```python
from build123d import *

# Parameters (mm, degrees)
F1_DEPTH = 50.8
F3_DEPTH = 45.72
F4_R     = 5.08


with BuildPart() as f1:
    # F0 (on Top) → F1 (new body)
    with BuildSketch(Plane.XY):
        Polygon((23.324189, 60.191778), (-32.517433, 55.764545), (-63.872765, 9.345472), (-47.130602, -44.110932), (5.101866, -64.350904), (53.492524, -36.133333), (61.602221, 19.293375), align=None)
    extrude(amount=F1_DEPTH)

    # F2 (on face) → F3 (cut)
    with BuildSketch(Plane.XY.offset(50.8)):
        Polygon((21.136437, 56.987757), (-31.37647, 52.056417), (-60.262255, 7.925533), (-43.769332, -42.173439), (5.68279, -60.514951), (50.855655, -33.287471), (57.733175, 19.006154), align=None)
    extrude(amount=-F3_DEPTH, mode=Mode.SUBTRACT)

    # F4
    f4_edges = [f1.edges().sort_by_distance(p)[0] for p in [
        (-63.872765, 9.345472, 25.4),
        (-32.517433, 55.764545, 25.4),
        (23.324189, 60.191778, 25.4),
        (61.602221, 19.293375, 25.4),
        (53.492524, -36.133333, 25.4),
        (-47.130602, -44.110932, 25.4),
        (5.101866, -64.350904, 25.4),
    ]]
    fillet(f4_edges, radius=F4_R)


solid = f1.part
```
Design review of the part built by this model. Coordinates are the model's own, in mm. A direction names the side the tool comes from. Give positions to 0.01 mm unless a question says otherwise; leave off trailing zeros. Write each loop counter-clockwise with the first axis right and the second up, starting at its lowest first coordinate (ties: lowest second). Pieces come first, ordered by that corner, then holes. Notation, with made-up numbers: (33, -10) - (53, -10) arc R34 ccw to (53, 27) - close; hole circle Ø4 at (63.5, 89). An arc over 180 degrees is marked (long way). Return JSON: item names as keys, results as strings. Group by question number.
(1) We need section A-A, the plane z = 11. Give the boundary of the cut face in (x, y), then the cut area to 3 significant figures.
(2) We need section B-B, the plane x = -28.5. Give the boundary of the cut face in (y, z), then the cut area to 3 significant figures.
(3) We need section C-C, the plane y = 49. Give the boundary of the cut face in (x, z).
(4) Machinability: for faces 5 (the flat face through (-47.995, 32.852, 25.044)), 6 (the flat face through (-2, -1, 5.08)), which of the approach directions +Z, -Z, +X, -X, +Y, -Y give a long, thin tool a straight path to every point of the face, cutting with its end or side? Answer none if there is none.
(5) To check wall thickness, follow probe 1 along X at (y, z) = (-27.5, 10); probe 2 along Z at (x, y) = (7.5, -21); probe 3 along Y at (x, z) = (41.5, 15.5). State the ranges of each line that lie inside material, in increasing order.
(6) Insertion check: pin 1 (6 mm diameter, centred on y = 8.5, z = 35, fed in from +X); pin 2 (10 mm diameter, centred on y = 10, z = 21.5, fed in from +X); pin 3 (12 mm diameter, centred on x = 8.5, z = 22.5, fed in from +Y). Each pin has a flat end and moves straight along its axis. Give the tip position at first contact, or say it passes through.
(7) Mouldability with a two-part tool opening along X and no side actions: class faces 1 (the flat face through (57.496, -8.774, 25.044)), 2 (the flat face through (-19.389, -51.216, 28.26)), 3 (the flat face through (27.953, -47.092, 28.26)), 4 (the flat face through (-21.35, -54.1, 25.04)) as +X half, -X half, draft (parallel to the pull), parting line (faces both ways), or undercut.
Reported:
{
 "1": {"outline": "(-63.14, 7.01) - (-47.86, -41.78) arc R5.08 ccw to (-44.85, -44.99) - (2.82, -63.47) arc R5.08 ccw to (7.22, -63.12) - (51.38, -37.37) arc R5.08 ccw to (53.85, -33.71) - (61.25, 16.87) arc R5.08 ccw to (59.93, 21.08) - (25, 58.41) arc R5.08 ccw to (20.89, 60) - (-30.08, 55.96) arc R5.08 ccw to (-33.89, 53.74) - (-62.5, 11.37) arc R5.08 ccw to start; hole (-60.26, 7.93) - (-43.77, -42.17) - (5.68, -60.51) - (50.86, -33.29) - (57.73, 19.01) - (21.14, 56.99) - (-31.38, 52.06) - close", "area": "1,290 mm2"},
 "2": {"outline": "(-51.33, 0) - (56.08, 0) - (56.08, 50.8) - (52.33, 50.8) - (52.33, 5.08) - (-47.84, 5.08) - (-47.84, 50.8) - (-51.33, 50.8) - close", "area": "877 mm2"},
 "3": {"outline": "(-37.09, 0) - (33.8, 0) - (33.8, 50.8) - (28.83, 50.8) - (28.83, 5.08) - (-33.38, 5.08) - (-33.38, 50.8) - (-37.09, 50.8) - close"},
 "4": {"face 5": "+Z, -Z, -X, +Y", "face 6": "+Z"},
 "5": {"probe 1": "x = -52.33 to -48.6, 51.62 to 54.76", "probe 2": "z = 0 to 5.08", "probe 3": "y = -43.13 to -38.93, 35.85 to 40.77"},
 "6": {"pin 1": "stops at x = 60.46", "pin 2": "stops at x = 60.97", "pin 3": "stops at y = 59.49"},
 "7": {"face 1": "+X half", "face 2": "undercut", "face 3": "undercut", "face 4": "-X half"}
}
